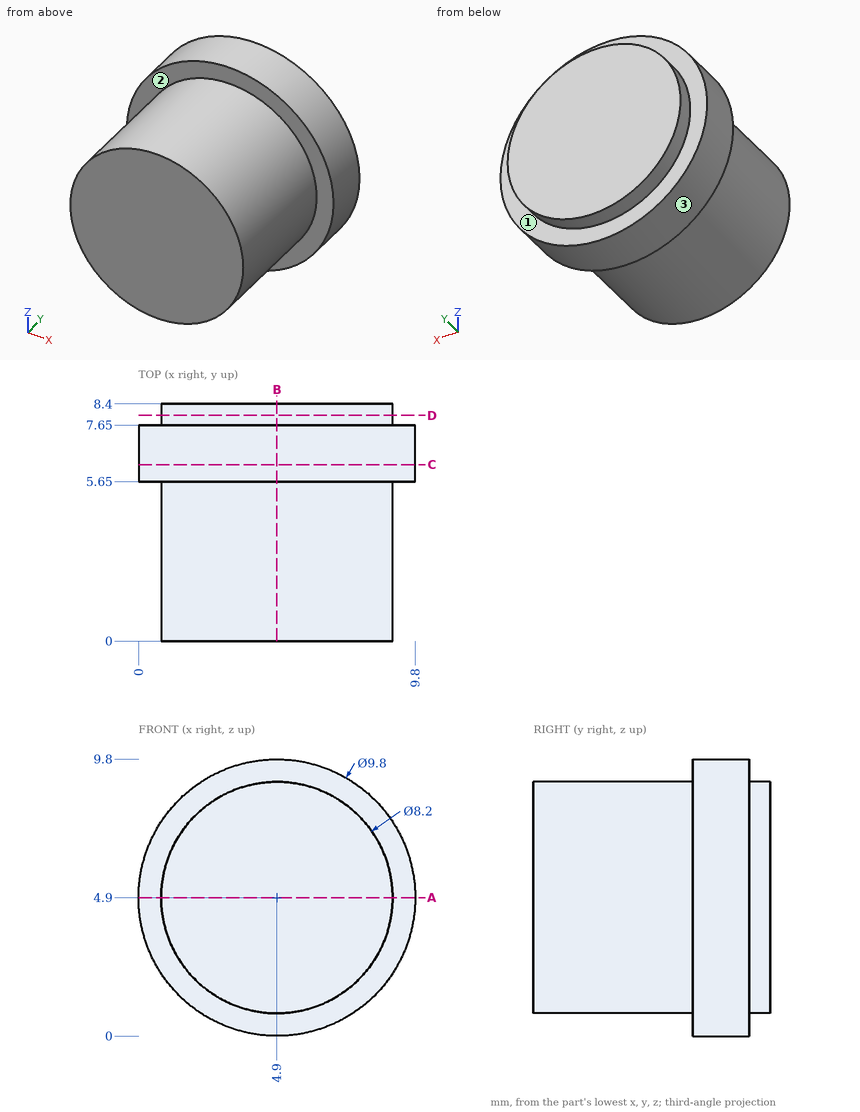
Answer from the drawing. Dimensions are ordinates in mm from the lowest x, y and z of the part. A direction names the side the tool comes from. Give positions to 0.01 mm unless a question says otherwise; leave off trailing zeros. Order: outer loops, then holes, each group sorted by start corner. A loop starts at its lowest first (then second) coordinate and runs counter-clockwise, first axis right, second up.
(1) Find section B-B (x = 4.9). Give the vertices of the cut face in (y, z), plus the area to 3 significant figures.
(2) Find section A-A (z = 4.9). Give the vertices of the cut face in (x, y), plus the area to 3 significant figures.
(3) Given pin 1 (1 mm diameter, centred on y = 5.5, z = 4, fed in from +X); pin 2 (2 mm diameter, centred on x = 1.5, y = 4.5, fed in from +Z); pin 3 (2 mm diameter, centred on x = 4, y = 2, fed in from +Z), each flat-ended and moving along its own axis, determine where each tip first touches the part or whether it passes through.
(4) Straight lines are drawn through the part: L1, parallel to Z at x = 5, y = 3; L2, parallel to Y at x = 6.5, z = 1; L3, parallel to Z at x = 8, y = 2.25. For each, find the intervals that lie inside material, in ascending order.
(5) For the marked faces 1, 2 and 3, determine the directions among +Z, -Z, +X, -X, +Y, -Y from which every point of the face is accessible in a straight line to the end or side of a thin tool.
(6) Find section D-D (y = 8). Give the vertices of the cut face in (x, z), plus the area to 3 significant figures.
(7) Find section C-C (y = 6.25). Give the vertices of the cut face in (x, z), plus the area to 3 significant figures.
Result sheet:
1. outline: (0, 0.8) - (5.65, 0.8) - (5.65, 0) - (7.65, 0) - (7.65, 0.8) - (8.4, 0.8) - (8.4, 9) - (7.65, 9) - (7.65, 9.8) - (5.65, 9.8) - (5.65, 9) - (0, 9) - close
1. area: 72.1 mm2
2. outline: (0, 5.65) - (0.8, 5.65) - (0.8, 0) - (9, 0) - (9, 5.65) - (9.8, 5.65) - (9.8, 7.65) - (9, 7.65) - (9, 8.4) - (0.8, 8.4) - (0.8, 7.65) - (0, 7.65) - close
2. area: 72.1 mm2
3. pin 1: stops at x = 9.78
3. pin 2: stops at z = 8.22
3. pin 3: stops at z = 9
4. L1: z = 0.8 to 9
4. L2: y = 5.65 to 7.65
4. L3: z = 2.22 to 7.58
5. face 1: +Y
5. face 2: -Y
5. face 3: +Y, -Y
6. outline: circle Ø8.2 at (4.9, 4.9)
6. area: 52.8 mm2
7. outline: circle Ø9.8 at (4.9, 4.9)
7. area: 75.4 mm2
